```python
from build123d import *

# Parameters (mm, degrees)
SKETCH1_R           = 6
BOSS_EXTRUDE1_DEPTH = 35
SKETCH2_R           = 2.921
CUT_EXTRUDE1_DEPTH  = 25.4
FILLET1_R           = 2.5


with BuildPart() as part:
    # Sketch1 → Boss-Extrude1 (new, symmetric)
    with BuildSketch(Plane.XY):
        Circle(SKETCH1_R)
    extrude(amount=BOSS_EXTRUDE1_DEPTH, both=True)

    # Sketch2 → Cut-Extrude1 (cut)
    with BuildSketch(Plane.XY.offset(35)):
        Circle(SKETCH2_R)
    cut_extrude1 = extrude(amount=-CUT_EXTRUDE1_DEPTH, mode=Mode.SUBTRACT)

    # Mirror1: Cut-Extrude1 across plane
    add(cut_extrude1.mirror(Plane.XY), mode=Mode.SUBTRACT)

    # Fillet1
    fillet1_edges = [part.edges().sort_by_distance(p)[0] for p in [
        (-2.921, 0, -9.6),
        (-2.921, 0, 9.6),
    ]]
    fillet(fillet1_edges, radius=FILLET1_R)


solid = part.part
```
The listing builds one solid part. Answer for the finished solid, in the listing's coordinates (mm). A direction names the side the tool comes from. Coordinates: 2 decimals unless noted, no trailing zeros. Loops run counter-clockwise (first coordinate to the right, second up) from the corner with the lowest first, then second, coordinate; pieces in that order, holes last. Notation, with made-up numbers: M -2.75,28.25 L 15.25,28.25 A35 cw 15.25,61.25 Z; hole C -31,17 d6. An arc over 180 degrees is marked long. Answer as CSV lines item,"result". Start each with the question number.
(1) The part is cut by section B-B (z = -7). Give the vertices of the cut face in (x, y), and give its area (3 significant figures).
(2) The mould has two halves that part along X. Classify faces 3 (the cylindrical face through (-6, 0, 0)), 4 (the flat face through (3, 1, -35)), 5 (the cylindrical face through (-0.633, -2.852, -23.71)): pulls with the +X half, pulls with the -X half, needs draft (parallel to the pull), parting line crosses it, or undercut.
(3) The part is cut by section C-C (x = -4). Give the vertices of the cut face in (y, z), and give its area (3 significant figures).
(4) Given pin 1 (1 mm diameter, centred on y = -3, z = -2.5, fed in from +X); pin 2 (1 mm diameter, centred on x = -1.5, z = 27, fed in from +Y); pin 3 (1 mm diameter, centred on x = -3, z = -12.5, fed in from +Y), each flat-ended and moving along its own axis, determine where each tip first touches the part or whether it passes through.
(5) The part is cut by section A-A (z = -18). Give the vertices of the cut face in (x, y), and give its area (3 significant figures).
(6) The part is cut by section D-D (y = 5). Give the vertices of the cut face in (x, z).
(7) For faces 1 (the cylindrical face through (-0.633, -2.852, 23.71)), 2 (the flat face through (3, 1, 35)), determine the directions among +Z, -Z, +X, -X, +Y, -Y from which every point of the face is accessible in a straight line to the end or side of a thin tool.
(8) Find the intervals of material crossed by L1, parallel to Y at x = 0, z = -26.5; L2, parallel to X at y = 0.5, z = 25.5; L3, parallel to Z at x = 0.5, y = -0.25, in increasing order. Write a range as [from, to].
Determined:
1,outline,"C 0,0 d12"
1,area,"113 mm2"
2,face 3,"parting line crosses it"
2,face 4,"needs draft"
2,face 5,"undercut"
3,outline,"M -4.47,-35 L 4.47,-35 L 4.47,35 L -4.47,35 Z"
3,area,"626 mm2"
4,pin 1,"x = 5.45"
4,pin 2,"y = 5.92"
4,pin 3,"y = 5.45"
5,outline,"C 0,0 d12; hole C 0,0 d5.84"
5,area,"86.3 mm2"
6,outline,"M -3.32,-35 L 3.32,-35 L 3.32,35 L -3.32,35 Z"
7,face 1,"+Z"
7,face 2,"+Z, +X, -X, +Y, -Y"
8,L1,"[-6, -2.92], [2.92, 6]"
8,L2,"[-5.98, -2.88], [2.88, 5.98]"
8,L3,"[-9.6, 9.6]"
